Work out the finished part from the listing and answer in its coordinate system (mm). Face numbers are marked on the shaded views. Coordinates: 2 decimals unless noted, no trailing zeros. Write each loop counter-clockwise with the first axis right and the second up, starting at its lowest first coordinate (ties: lowest second). Pieces come first, ordered by that corner, then holes. Notation, with made-up numbers: M -7,31 L 48,31 A26 cw 48,69 Z; hole C 47,6 d11. An arc over 180 degrees is marked long. Answer as CSV lines item,"result". Start each with the question number.
(1) A cutting plane is placed at C-C on y = 233.5. Give the vertices of the cut face in (x, z).
(2) Find the intervals of material crossed by L1, parallel to Y at x = -132, z = 25; L2, parallel to X at y = 122, z = 51; L3, parallel to Z at x = -96.5, y = -208, in increasing order. Write a range as [from, to].
(3) A cutting plane is placed at D-D on y = 123. Give the vertices of the cut face in (x, z), then the cut area to 3 significant figures.
(4) Flat-ended cylindrical pins translate along their axes: P1, Ø12, axis at x = -58, y = 262, coming from the +Z side; P2, Ø4, axis at x = -130, z = 80, coming from the +Y side. Find the tip coordinate at first contact, or state that the pin passes through.
(5) The mould has two halves that part along X. Classify the marked faces 1, 2, 3 and 4: released by +X, released by -X, zero draft, split by the parting line, or undercut.
(6) A cutting plane is placed at B-B on z = 63.5. Give the vertices of the cut face in (x, y).
(7) A cutting plane is placed at A-A on x = -85. Give the vertices of the cut face in (y, z).
from build123d import *

# Parameters (mm, degrees)
F0_W      = 101.6
F0_H      = 609.6
F0_W_2    = 76.2
F0_H_2    = 558.8
F1_DEPTH  = 127
F2_W      = 76.2
F2_H      = 558.8
F3_DEPTH  = 19.05
F4_W      = 76.2
F4_H      = 25.4
F5_DEPTH  = 6.35
F6_W      = 101.6
F6_H      = 101.6
F7_DEPTH  = 25.4
F8_W      = 101.6
F8_H      = 101.6
F9_DEPTH  = 25.4
F10_DEPTH = 6.35
F11_R     = 6.35
F12_DEPTH = 6.35
F13_R     = 6.35
F14_DEPTH = 12.7
F15_DEPTH = 127
F16_W     = 25.4
F16_H     = 25.4
F17_DEPTH = 6.35
F18_R     = 6.35
F19_DEPTH = 6.35
F20_R     = 5.08
F21_R     = 31.75
F22_DEPTH = 12.7
F23_R     = 3.175
F24_DEPTH = 101.6


with BuildPart() as f1:
    # F0 (on Top) → F1 (new body)
    with BuildSketch(Plane.XY):
        with Locations((-88.1464483801, 27.3514616579)):
            Rectangle(F0_W, F0_H)
        with Locations((-88.1464483801, 27.3514616579)):
            Rectangle(F0_W_2, F0_H_2, mode=Mode.SUBTRACT)
    extrude(amount=F1_DEPTH)

    # F2 (on face) → F3 (join)
    with BuildSketch(Plane(origin=(0, 0, 0), x_dir=(1, 0, 0), z_dir=(0, 0, -1))):
        with Locations((-88.1464483801, -27.3514616579)):
            Rectangle(F2_W, F2_H)
    extrude(amount=-F3_DEPTH)

    # F4 (on face) → F5 (join)
    with BuildSketch(Plane.XY.offset(127)):
        with Locations((-88.1464483801, 65.4514616579)):
            Rectangle(F4_W, F4_H)
        with Locations((-88.1464483801, -86.9485383421)):
            Rectangle(F4_W, F4_H)
    extrude(amount=-F5_DEPTH)

    # F6 (on face) → F7 (cut)
    with BuildSketch(Plane.XZ.offset(277.4485383421)):
        with Locations((-88.1464483801, 63.5)):
            Rectangle(F6_W, F6_H)
    extrude(amount=-F7_DEPTH, mode=Mode.SUBTRACT)

    # F8 (on face) → F9 (cut)
    with BuildSketch(Plane(origin=(0, 332.1514616579, 0), x_dir=(-1, 0, 0), z_dir=(0, 1, 0))):
        with Locations((88.1464483801, 63.5)):
            Rectangle(F8_W, F8_H)
    extrude(amount=-F9_DEPTH, mode=Mode.SUBTRACT)

    # F10 (cut): a face of the model
    f10_faces = [f1.faces().sort_by_distance(p)[0] for p in [
        (-88.1464483801, 27.3514616579, 19.05),
    ]]
    extrude(f10_faces, amount=-F10_DEPTH, mode=Mode.SUBTRACT)

    # F11 (on face) → F12 (cut)
    with BuildSketch(Plane.XY.offset(127)):
        with Locations((-113.5464483801, 65.4514616579)):
            Circle(F11_R)
        with Locations((-113.5464483801, -86.9485383421)):
            Circle(F11_R)
    extrude(amount=-F12_DEPTH, mode=Mode.SUBTRACT)

    # F13 (on face) → F14 (cut)
    with BuildSketch(Plane.XY.offset(127)):
        with Locations((-119.8964483801, -264.7485383421)):
            Circle(F13_R)
        with Locations((-56.3964483801, -264.7485383421)):
            Circle(F13_R)
        with Locations((-119.8964483801, 319.4514616579)):
            Circle(F13_R)
        with Locations((-56.3964483801, 319.4514616579)):
            Circle(F13_R)
    extrude(amount=-F14_DEPTH, mode=Mode.SUBTRACT)

    # F13 (on face) → F15 (cut)
    with BuildSketch(Plane.XY.offset(127)):
        with Locations((-119.8964483801, 319.4514616579)):
            Circle(F13_R)
        with Locations((-56.3964483801, 319.4514616579)):
            Circle(F13_R)
        with Locations((-119.8964483801, -264.7485383421)):
            Circle(F13_R)
        with Locations((-56.3964483801, -264.7485383421)):
            Circle(F13_R)
    extrude(amount=-F15_DEPTH, mode=Mode.SUBTRACT)

    # F16 (on face) → F17 (join)
    with BuildSketch(Plane.XY.offset(127)):
        with Locations((-113.5464483801, -175.8485383421)):
            Rectangle(F16_W, F16_H)
        with Locations((-113.5464483801, 192.4514616579)):
            Rectangle(F16_W, F16_H)
    extrude(amount=-F17_DEPTH)

    # F18 (on face) → F19 (cut)
    with BuildSketch(Plane.XY.offset(127)):
        with Locations((-113.5464483801, 192.4514616579)):
            Circle(F18_R)
        with Locations((-113.5464483801, -175.8485383421)):
            Circle(F18_R)
    extrude(amount=-F19_DEPTH, mode=Mode.SUBTRACT)

    # F20
    f20_edges = [f1.edges().sort_by_distance(p)[0] for p in [
        (-126.246448, -99.648538, 123.825),
        (-50.046448, -99.648538, 123.825),
        (-100.846448, -163.148538, 123.825),
        (-100.846448, -188.548538, 123.825),
        (-126.246448, -188.548538, 123.825),
        (-126.246448, -163.148538, 123.825),
        (-50.046448, -252.048538, 120.65),
        (-50.046448, -74.248538, 123.825),
        (-126.246448, -74.248538, 123.825),
        (-50.046448, 52.751462, 123.825),
        (-126.246448, 52.751462, 123.825),
        (-126.246448, 179.751462, 123.825),
        (-126.246448, 78.151462, 123.825),
        (-50.046448, 78.151462, 123.825),
        (-100.846448, 179.751462, 123.825),
        (-126.246448, 205.151462, 123.825),
        (-100.846448, 205.151462, 123.825),
        (-126.246448, 306.751462, 120.65),
        (-126.246448, -252.048538, 120.65),
        (-50.046448, 306.751462, 120.65),
    ]]
    fillet(f20_edges, radius=F20_R)

    # F21 (on face) → F22 (cut)
    with BuildSketch(Plane(origin=(-138.9464483801, 0, 0), x_dir=(0, -1, 0), z_dir=(-1, 0, 0))):
        with Locations((-230.5514616579, 63.5)):
            Circle(F21_R)
        with Locations((175.8485383421, 63.5)):
            Circle(F21_R)
    extrude(amount=-F22_DEPTH, mode=Mode.SUBTRACT)

    # F23 (on face) → F24 (cut)
    with BuildSketch(Plane(origin=(-138.9464483801, 0, 0), x_dir=(0, -1, 0), z_dir=(-1, 0, 0))):
        with Locations((137.7485383421, 101.6)):
            Circle(F23_R)
        with Locations((137.7485383421, 25.4)):
            Circle(F23_R)
        with Locations((213.9485383421, 25.4)):
            Circle(F23_R)
        with Locations((213.9485383421, 101.6)):
            Circle(F23_R)
        with Locations((-192.4514616579, 25.4)):
            Circle(F23_R)
        with Locations((-268.6514616579, 25.4)):
            Circle(F23_R)
        with Locations((-268.6514616579, 101.6)):
            Circle(F23_R)
        with Locations((-192.4514616579, 101.6)):
            Circle(F23_R)
    extrude(amount=-F24_DEPTH, mode=Mode.SUBTRACT)


solid = f1.part
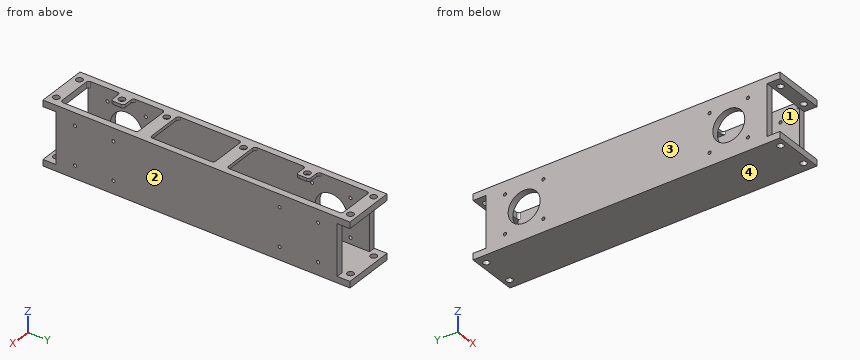
Here are the results:
1,outline,"M -138.95,0 L -37.35,0 L -37.35,127 L -50.05,127 L -50.05,12.7 L -126.25,12.7 L -126.25,31.89 L -138.95,31.89 Z; M -138.95,95.11 L -126.25,95.11 L -126.25,127 L -138.95,127 Z"
2,L1,"y = [-252.05, -217.1], [-210.8, -140.9], [-134.6, 189.3], [195.6, 265.5], [271.8, 306.75]"
2,L2,"x = [-138.95, -126.25], [-50.05, -37.35]"
2,L3,"z = [0, 12.7]"
3,outline,"M -138.95,0 L -37.35,0 L -37.35,127 L -50.05,127 L -50.05,12.7 L -126.25,12.7 L -126.25,127 L -138.95,127 Z"
3,area,"4,190 mm^2"
4,P1,"stops at z = 12.7"
4,P2,"stops at y = 306.75"
5,face 1,"undercut"
5,face 2,"released by +X"
5,face 3,"released by -X"
5,face 4,"zero draft"
6,outline,"M -138.95,-252.05 L -126.25,-252.05 L -126.25,-207.6 L -138.95,-207.6 Z; M -138.95,-144.1 L -126.25,-144.1 L -126.25,198.8 L -138.95,198.8 Z; M -138.95,262.3 L -126.25,262.3 L -126.25,306.75 L -138.95,306.75 Z; M -50.05,-252.05 L -37.35,-252.05 L -37.35,306.75 L -50.05,306.75 Z"
7,outline,"M -277.45,0 L 332.15,0 L 332.15,12.7 L -277.45,12.7 Z; M -277.45,114.3 L -252.05,114.3 L -252.05,127 L -277.45,127 Z; M -99.65,120.65 L -74.25,120.65 L -74.25,127 L -99.65,127 Z; M 52.75,120.65 L 78.15,120.65 L 78.15,127 L 52.75,127 Z; M 306.75,114.3 L 332.15,114.3 L 332.15,127 L 306.75,127 Z"
